Geometry check sheet. Reference: the model listing, model coordinates, mm. Face numbers are marked on the shaded views. A direction names the side the tool comes from. Give positions to 0.01 mm unless a question says otherwise; leave off trailing zeros. Write each loop counter-clockwise with the first axis right and the second up, starting at its lowest first coordinate (ties: lowest second). Pieces come first, ordered by that corner, then holes. Notation, with made-up numbers: (77, 75.25) -> (88, 75.25) arc R26 ccw to (88, 96.25) -> close; hole circle Ø7 at (-30, 43). An arc over 180 degrees is marked (long way). One line per item, written item: value.
from build123d import *

# Parameters (mm, degrees)
F3_DEPTH = 6
F4_DEPTH = 50
F1_W     = 5
F1_H     = 5
F6_DEPTH = 54
F7_DEPTH = 54
F2_R     = 20
F8_DEPTH = 50
F9_DEPTH = 30


with BuildPart() as f3:
    # F2 (on Top) → F3 (new body)
    with BuildSketch(Plane.XY):
        with BuildLine():
            Line((-45.5, 75), (-99.5, 75))
            Line((-99.5, 75), (-99.5, 21))
            Line((-99.5, 21), (-69.5, 21))
            ThreePointArc((-69.5, 21), (-86.470563, 61.970563), (-45.5, 45))
            Line((-45.5, 45), (-45.5, 75))
        make_face()
        with BuildLine():
            Line((-20, 75), (-45.5, 75))
            Line((-45.5, 75), (-45.5, 45))
            ThreePointArc((-45.5, 45), (-52.529437, 28.029437), (-69.5, 21))
            Line((-69.5, 21), (-99.5, 21))
            Line((-99.5, 21), (-99.5, -75))
            Line((-99.5, -75), (99.5, -75))
            Line((99.5, -75), (99.5, 75))
            Line((99.5, 75), (20, 75))
            Line((20, 75), (-20, 75))
        make_face()
    extrude(amount=F3_DEPTH)

    # F1 (on Top) → F4 (join)
    with BuildSketch(Plane.XY):
        Polygon((99.5, 75), (-99.5, 75), (-99.5, -75), (-95.5, -75), (-95.5, -70), (-95.5, 66), (-95.5, 71), (-90.5, 71), (0, 71), (90.394951, 71), (95.394951, 71), (95.394951, 66), (95.394951, -70), (95.394951, -75), (99.5, -75), align=None)
        Polygon((-95.5, -70), (-95.5, -75), (-90.5, -75), (-90.5, -71.581401), (-90.5, -70), align=None)
        Polygon((90.394951, -75), (95.394951, -75), (95.394951, -70), (90.394951, -70), (90.394951, -71.581401), align=None)
        Polygon((-90.5, -71.581401), (-90.5, -75), (0, -75), (90.394951, -75), (90.394951, -71.581401), align=None)
    extrude(amount=F4_DEPTH)

    # F1 (on Top) → F6 (join)
    with BuildSketch(Plane.XY):
        with Locations((-93, 68.5)):
            Rectangle(F1_W, F1_H)
    extrude(amount=F6_DEPTH)

    # F1 (on Top) → F7 (join)
    with BuildSketch(Plane.XY):
        with Locations((92.894951, 68.5)):
            Rectangle(F1_W, F1_H)
        Polygon((90.394951, -75), (95.394951, -75), (95.394951, -70), (90.394951, -70), (90.394951, -71.581401), align=None)
        Polygon((-95.5, -70), (-95.5, -75), (-90.5, -75), (-90.5, -71.581401), (-90.5, -70), align=None)
    extrude(amount=F7_DEPTH)

    # F2 (on Top) → F8 (join)
    with BuildSketch(Plane.XY):
        with BuildLine():
            ThreePointArc((-69.5, 21), (-52.529437, 28.029437), (-45.5, 45))
            ThreePointArc((-45.5, 45), (-86.470563, 61.970563), (-69.5, 21))
        make_face()
        with Locations((-69.5, 45)):
            Circle(F2_R, mode=Mode.SUBTRACT)
        with BuildLine():
            Line((-45.5, 75), (-99.5, 75))
            Line((-99.5, 75), (-99.5, 21))
            Line((-99.5, 21), (-69.5, 21))
            ThreePointArc((-69.5, 21), (-86.470563, 61.970563), (-45.5, 45))
            Line((-45.5, 45), (-45.5, 75))
        make_face()
    extrude(amount=F8_DEPTH)

    # F1 (on Top) → F9 (cut)
    with BuildSketch(Plane.XY):
        Polygon((-95.5, 66), (-95.5, -70), (-90.5, -70), (-90.5, -71.581401), (90.394951, -71.581401), (90.394951, -70), (95.394951, -70), (95.394951, 66), (90.394951, 66), (90.394951, 71), (0, 71), (-90.5, 71), (-90.5, 66), align=None)
        with Locations((-93, 68.5)):
            Rectangle(F1_W, F1_H)
        with Locations((92.894951, 68.5)):
            Rectangle(F1_W, F1_H)
    extrude(amount=F9_DEPTH, mode=Mode.SUBTRACT)


solid = f3.part
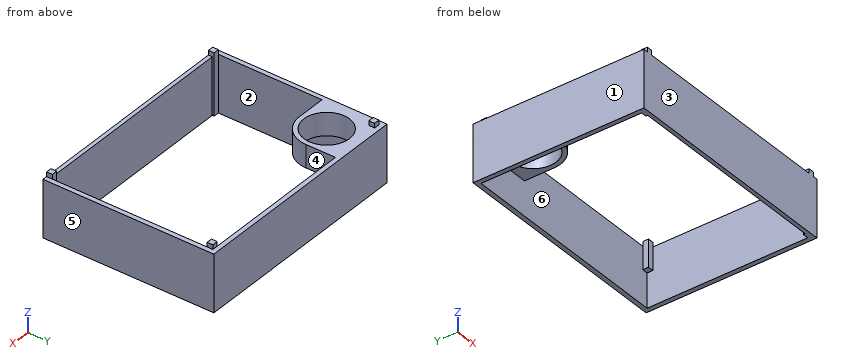
1) Sectioned sample at A-A on x = -25. Record the cut outline in (y, z), plus the area to 3 significant figures.
Verdict:
outline: (-75, 0) -> (-71.58, 0) -> (-71.58, 50) -> (-75, 50) -> close; (71, 0) -> (75, 0) -> (75, 50) -> (71, 50) -> close
area: 371 mm^2
2) Mould release check, pull along Y, two halves, no side actions. Record for the marked faces 1, 2 and 3: released by +Y, released by -Y, zero draft, split by the parting line, or undercut.
Verdict:
face 1: zero draft
face 2: undercut
face 3: released by -Y
3) Sectioned sample at C-C on y = 38. Record the cut outline in (x, z) (3 decimals), plus the area to 3 significant figures.
Verdict:
outline: (-99.5, 0) -> (-95.5, 0) -> (-95.5, 30) -> (-88.235, 30) -> (-88.235, 50) -> (-99.5, 50) -> close; (-50.765, 30) -> (-46.544, 30) -> (-46.544, 50) -> (-50.765, 50) -> close; (95.395, 0) -> (99.5, 0) -> (99.5, 50) -> (95.395, 50) -> close
area: 635 mm^2
4) Scan lines: probe 1 along X at (y, z) = (45, 44.5); probe 2 along Y at (x, z) = (-69.5, 40.25); probe 3 along Y at (x, z) = (-65.5, 43.5). Record each from-to range of solid material in increasing order.
Verdict:
probe 1: -99.5 to -89.5, -49.5 to -45.5, 95.39 to 99.5
probe 2: -75 to -71.58, 21 to 25, 65 to 75
probe 3: -75 to -71.58, 21.34 to 25.4, 64.6 to 75
5) Depth check by flat-ended pin: pin 1 Ø2 at (y, z) = (68.5, 52.5) entering from -X; pin 2 Ø3 at (x, z) = (93, 52.5) entering from +Y; pin 3 Ø1.5 at (x, y) = (92.5, 68.5) entering from -Z. Enter the tip coordinate at first touch or a pass-through.
Verdict:
pin 1: x = -95.5
pin 2: y = 71
pin 3: z = 30
6) Sectioned sample at D-D on x = -83. Record the cut outline in (y, z).
Verdict:
outline: (-75, 0) -> (-71.58, 0) -> (-71.58, 50) -> (-75, 50) -> close; (21, 30) -> (30.24, 30) -> (30.24, 50) -> (21, 50) -> close; (59.76, 30) -> (71, 30) -> (71, 0) -> (75, 0) -> (75, 50) -> (59.76, 50) -> close
7) Sectioned sample at B-B on z = 15. Record the cut outline in (x, y).
Verdict:
outline: (-99.5, -75) -> (99.5, -75) -> (99.5, 75) -> (-99.5, 75) -> close; hole (-95.5, -70) -> (-90.5, -70) -> (-90.5, -71.58) -> (90.39, -71.58) -> (90.39, -70) -> (95.39, -70) -> (95.39, 71) -> (-95.5, 71) -> close
8) Tool access check on the marked faces 4, 5 and 6. Record the directions out of +Z, -Z, +X, -X, +Y, -Y that give a thin tool (end or side, any length) a straight path to the whole face; none if there is none.
Verdict:
face 4: +Z, -Z
face 5: +Z, -Z, +X, +Y, -Y
face 6: -Z
